Check sheet for the drawn part. Datum: minimum x, y, z corner. Units: mm. A direction names the side the tool comes from. Give positions to 0.01 mm unless a question says otherwise; leave off trailing zeros. Order: outer loops, then holes, each group sorted by start corner. A loop starts at its lowest first (then second) coordinate and runs counter-clockwise, first axis right, second up.
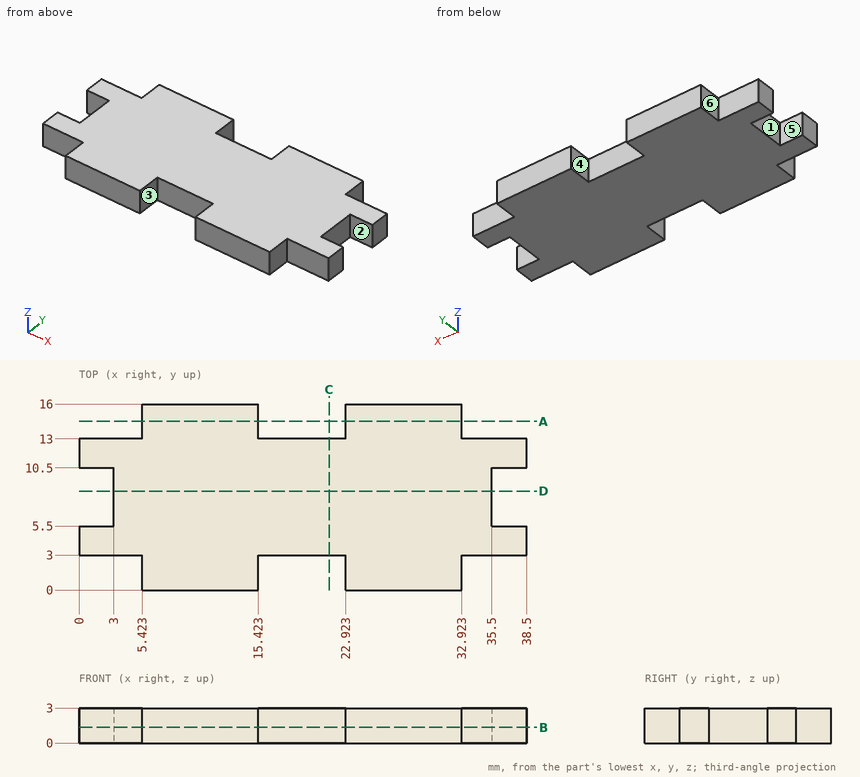
Item 1: Sectioned sample at D-D (y = 8.5). Enter the section's corners in (x, z).
Reported:
outline: (3, 0) - (35.5, 0) - (35.5, 3) - (3, 3) - close
Item 2: Scan lines: L1, parallel to X at y = 1.5, z = 0.4; L2, parallel to Y at x = 21, z = 0.95; L3, parallel to X at y = 7.5, z = 0.4. Record each from-to range of solid material in increasing order.
Reported:
L1: x = 5.42 to 15.42, 22.92 to 32.92
L2: y = 3 to 13
L3: x = 3 to 35.5
Item 3: Sectioned sample at A-A (y = 14.5). Enter the section's corners in (x, z), and give its area (3 significant figures).
Reported:
outline: (5.42, 0) - (15.42, 0) - (15.42, 3) - (5.42, 3) - close; (22.92, 0) - (32.92, 0) - (32.92, 3) - (22.92, 3) - close
area: 60.0 mm2
Item 4: Set-up check for the marked faces 1, 2 and 3: record each of +Z, -Z, +X, -X, +Y, -Y from which the full face is reachable in a straight line by a thin tool's end or side.
Reported:
face 1: +Z, -Z, -X
face 2: +Z, -Z, +X
face 3: +Z, -Z, -Y
Item 5: Sectioned sample at C-C (x = 21.5). Enter the section's corners in (y, z), and give its area (3 significant figures).
Reported:
outline: (3, 0) - (13, 0) - (13, 3) - (3, 3) - close
area: 30.0 mm2
Item 6: Sectioned sample at B-B (z = 1.35). Enter the section's corners in (x, y).
Reported:
outline: (0, 3) - (5.42, 3) - (5.42, 0) - (15.42, 0) - (15.42, 3) - (22.92, 3) - (22.92, 0) - (32.92, 0) - (32.92, 3) - (38.5, 3) - (38.5, 5.5) - (35.5, 5.5) - (35.5, 10.5) - (38.5, 10.5) - (38.5, 13) - (32.92, 13) - (32.92, 16) - (22.92, 16) - (22.92, 13) - (15.42, 13) - (15.42, 16) - (5.42, 16) - (5.42, 13) - (0, 13) - (0, 10.5) - (3, 10.5) - (3, 5.5) - (0, 5.5) - close
Item 7: Draft check along X on the marked faces 4, 5 and 6. Enter one of: released by +X, released by -X, zero draft, split by the parting line, or undercut.
Reported:
face 4: undercut
face 5: zero draft
face 6: released by -X
Item 8: Gauge pin test, flat ends, axial feed: pin 1 (1.5 mm diameter, centred on y = 15, z = 2, fed in from -X); pin 2 (1.5 mm diameter, centred on x = 3, z = 2, fed in from -Y); pin 3 (0.9 mm diameter, centred on y = 2, z = 1.5, fed in from +X). Record the tip position at first contact, or that the pin passes through.
Reported:
pin 1: stops at x = 5.42
pin 2: stops at y = 3
pin 3: stops at x = 32.92
